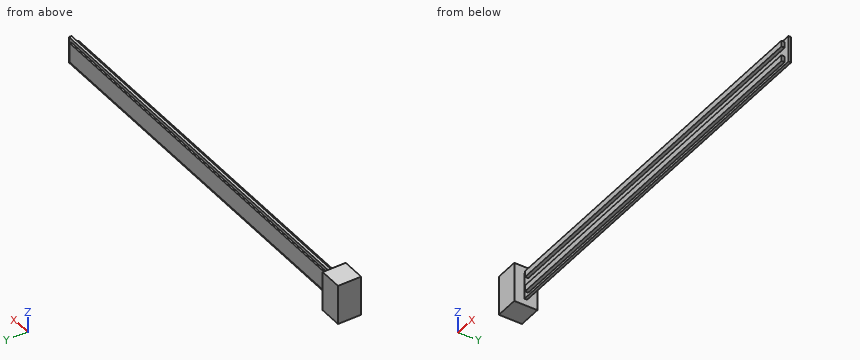
from build123d import *

# Parameters (mm, degrees)
SKETCH1_W           = 35
SKETCH1_H           = 35
BOSS_EXTRUDE1_DEPTH = 60
SKETCH2_W           = 40
SKETCH2_H           = 4
BOSS_EXTRUDE2_DEPTH = 600
SKETCH3_W           = 590
SKETCH3_H           = 30
BOSS_EXTRUDE3_DEPTH = 2.6
SKETCH4_W           = 582.794141244
SKETCH4_H           = 9.091842743
BOSS_EXTRUDE6_DEPTH = 5


with BuildPart() as part:
    # Sketch1 → Boss-Extrude1 (new body)
    with BuildSketch(Plane.XY):
        Rectangle(SKETCH1_W, SKETCH1_H)
    extrude(amount=BOSS_EXTRUDE1_DEPTH)

    # Sketch2 → Boss-Extrude2 (add)
    with BuildSketch(Plane(origin=(17.5, 0, 0), x_dir=(0, 0, -1), z_dir=(1, 0, 0))):
        with Locations((-30, 0)):
            Rectangle(SKETCH2_W, SKETCH2_H)
    extrude(amount=BOSS_EXTRUDE2_DEPTH)

    # Sketch3 → Boss-Extrude3 (add)
    with BuildSketch(Plane(origin=(0, 2, 0), x_dir=(1, 0, 0), z_dir=(0, 1, 0))):
        with Locations((317.5, -30)):
            Rectangle(SKETCH3_W, SKETCH3_H)
    extrude(amount=BOSS_EXTRUDE3_DEPTH)

    # Sketch4 → Boss-Extrude6 (add)
    with BuildSketch(Plane.XZ.offset(2)):
        with Locations((317.5, 41.36480343)):
            Rectangle(SKETCH4_W, SKETCH4_H)
    boss_extrude6 = extrude(amount=BOSS_EXTRUDE6_DEPTH)

    # Mirror1: Boss-Extrude6 across plane
    add(boss_extrude6.mirror(Plane.XY.offset(30)))


solid = part.part
Check sheet for the modelled part. Datum: model origin and axes. Units: mm. Give positions to 0.01 mm unless a question says otherwise; leave off trailing zeros. Loops run counter-clockwise (first coordinate to the right, second up) from the corner with the lowest first, then second, coordinate; pieces in that order, holes last. Notation, with made-up numbers: M 1.5,-1.75 L 51.5,-1.75 A16 cw 51.5,2.25 Z; hole C 40,15.5 d3. An arc over 180 degrees is marked long. Use a Markdown table: item, result. Add a question column.
Q1. Scan lines: line 1 along Z through (x, y) = (382, -2.5); line 2 along X through (y, z) = (12, 4.5); line 3 along Y through (x, z) = (96, 40). Record each from-to range of solid material in increasing order. Write a range as [from, to].
Q2. Go/stop test with flat-tipped pins: pin 1 (9 mm diameter, centred on x = 366, z = 27, fed in from +Y); pin 2 (2.5 mm diameter, centred on y = -5.5, z = 20, fed in from +X); pin 3 (2.5 mm diameter, centred on x = 173.5, y = -5, fed in from +Z). Record where each tip stops, or that it passes through.
Q3. Sectioned sample at A-A, the plane x = 415. Record the cut outline in (y, z).
Verdict:
| question | item | result |
|---|---|---|
| 1 | line 1 | [14.09, 23.18], [36.82, 45.91] |
| 1 | line 2 | [-17.5, 17.5] |
| 1 | line 3 | [-7, 4.6] |
| 2 | pin 1 | y = 4.6 |
| 2 | pin 2 | x = 608.9 |
| 2 | pin 3 | z = 45.91 |
| 3 | outline | M -7,14.09 L -2,14.09 L -2,10 L 2,10 L 2,15 L 4.6,15 L 4.6,45 L 2,45 L 2,50 L -2,50 L -2,45.91 L -7,45.91 L -7,36.82 L -2,36.82 L -2,23.18 L -7,23.18 Z |
